For this review, take the finished solid that the model builds, in its own axes (mm). Face numbers are marked on the shaded views. A direction names the side the tool comes from. Give positions to 0.01 mm unless a question says otherwise; leave off trailing zeros. Write each loop counter-clockwise with the first axis right and the second up, starting at its lowest first coordinate (ties: lowest second). Pieces come first, ordered by that corner, then holes. Notation, with made-up numbers: (-5.75, 75.5) -> (20.25, 75.5) arc R22 cw to (20.25, 91.5) -> close; hole circle Ø3 at (61, 6). An arc over 180 degrees is marked (long way). Write item = value, one per line.
Autodesk Inventor part; units mm, degrees
ref_plane "YZ Plane" through (0, 0, 0) normal (1, 0, 0) x (0, 1, 0)
ref_plane "XZ Plane" through (0, 0, 0) normal (0, 1, 0) x (-1, 0, 0)
ref_plane "XY Plane" through (0, 0, 0) normal (0, 0, 1) x (1, 0, 0)
sketch "Sketch1" plane through (0, 0, 0) normal (0, 1, 0) x (-1, 0, 0)
  circle A0 centre (0, 0) radius 5
  dimension "d0" = 10
extrude "Extrusion1" add sketch "Sketch1" against normal blind 1.5
sketch "Sketch2" plane through (0, -1.5, 0) normal (0, -1, 0) x (1, 0, 0)
  circle A0 centre (0, 0) radius 2.875
  dimension "d3" = 5.75
extrude "Extrusion2" add sketch "Sketch2" along normal blind 6.75
sketch "Sketch3" plane through (0, -8.25, 0) normal (0, -1, 0) x (1, 0, 0)
  circle A0 centre (0, 0) radius 2
  dimension "d6" = 4
extrude "Extrusion3" add sketch "Sketch3" along normal blind 0.75
sketch "Sketch4" plane through (0, 0, 0) normal (1, 0, 0) x (0, 1, 0)
  line L0 (0, -5) -> (0, 5)
  arc A0 (0, -5) -> (0, 5) centre (-4.1533, 0) ccw
  line L1 (0, 5) -> (-0.75, 5)
  line L2 (0, 5) -> (-1.5, 5)
  line L3 (0, -5) -> (-1.5, -5)
  line L4 (-0.75, -5) -> (0, -5)
  line L5 (-4.1533, 5) -> (-4.1533, -5) construction
  point P0 (0, 0)
  dimension "d9" = 6.5
revolve "Revolution1" add sketch "Sketch4" angle 101 mid plane about axis through (0, -4.1533, 5) along (0, 0, -1)
sketch "Sketch5" plane through (0, 0, 0) normal (0, 1, 0) x (-1, 0, 0)
  circle A0 centre (0, 0) radius 5
  circle A1 centre (0, 0) radius 8.973
extrude "Extrusion4" cut sketch "Sketch5" against normal mid plane 100
sketch "Sketch6" plane through (0, 0, 0) normal (1, 0, 0) x (0, 1, 0)
  line L0 (-8.25, 2.875) -> (-8.25, -2.875)
  line L1 (0.85, 0.75) -> (5.85, 0.75)
  line L2 (5.85, 0.75) -> (5.85, -0.75)
  line L3 (5.85, -0.75) -> (0.85, -0.75)
  line L4 (0.85, -0.75) -> (0.85, 0.75)
  point P0 (0, 0)
  dimension "d14" = 1.5
  dimension "d15" = 5
extrude "Extrusion5" cut sketch "Sketch6" against normal mid plane 10
properties part number "1 Prisionero" material "Steel"
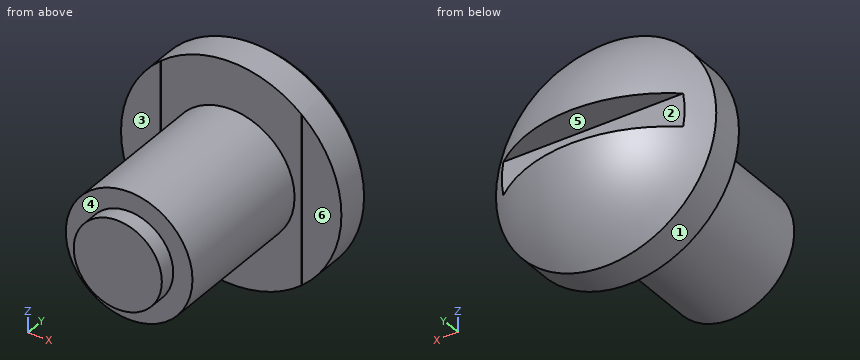
(1) The part is to be moulded in two halves that separate along Z. For the marked faces 1, 2 and 3, say which applies: released by +Z, released by -Z, zero draft, split by the parting line, or undercut.
Answers below:
face_1 = split by the parting line
face_2 = undercut
face_3 = zero draft
(2) For pin 1 (1.6 mm diameter, centred on x = 0.5, y = 1.5, fed in from -Z); pin 2 (3 mm diameter, centred on y = -6, z = -3.5, fed in from -X); pin 3 (1 mm diameter, centred on y = -5.5, z = 0.5, fed in from +X) (3 decimals), all flat-tipped, find the tip position at first contact; note any pin that passes through.
Answers below:
pin_1 = -4.3
pin_2 = -2.07
pin_3 = 2.875
(3) Tool access review of the marked faces 4, 5 and 6: name each direction out of +Z, -Z, +X, -X, +Y, -Y from which nothing blocks a thin tool from reaching the whole face with its end or side.
Answers below:
face_4 = -Y
face_5 = +X, -X, +Y
face_6 = +Z, -Z, +X, -Y
(4) Take a section at A-A (x = 0). Write out the cut boundary in (y, z) (3 decimals).
Answers below:
outline = (-9, -2) -> (-8.25, -2) -> (-8.25, -2.875) -> (-1.5, -2.875) -> (-1.5, -5) -> (0, -5) arc R6.5 ccw to (2.303, -0.75) -> (0.85, -0.75) -> (0.85, 0.75) -> (2.303, 0.75) arc R6.5 ccw to (0, 5) -> (-1.5, 5) -> (-1.5, 2.875) -> (-8.25, 2.875) -> (-8.25, 2) -> (-9, 2) -> close
(5) To check wall thickness, follow probe 1 along Y at (x, z) = (-4, 0.25); probe 2 along Y at (x, z) = (2.5, -0.25); probe 3 along Z at (x, y) = (-1.5, -7). State the ranges of each line that lie inside material, in increasing order.
Answers below:
probe_1 = -1.5 to 0.85
probe_2 = -8.25 to 0.85
probe_3 = -2.45 to 2.45
(6) Take a section at B-B (z = 0). Write out the cut boundary in (x, y) (3 decimals), plus the area to 3 significant figures.
Answers below:
outline = (-5, -1.5) -> (-3.219, -1.5) -> (-3.205, -1.511) arc R4.153 cw to (-3.195, -1.5) -> (-2.875, -1.5) -> (-2.875, -8.25) -> (-2, -8.25) -> (-2, -9) -> (2, -9) -> (2, -8.25) -> (2.875, -8.25) -> (2.875, -1.5) -> (3.195, -1.5) arc R4.153 cw to (3.205, -1.511) -> (3.219, -1.5) -> (5, -1.5) -> (5, 0) arc R6.5 ccw to (4.149, 0.85) -> (-4.149, 0.85) arc R6.5 ccw to (-5, 0) -> close
area = 64.6 mm^2
(7) Take a section at C-C (y = -5.5). Write out the cut boundary in (x, z) (3 decimals), plus the area to 3 significant figures.
Answers below:
outline = circle Ø5.75 at (0, 0)
area = 26.0 mm^2
